from build123d import *

# Parameters (mm, degrees)
F0_W     = 55
F0_H     = 60
F1_DEPTH = 45
F2_W     = 55
F2_H     = 25
F3_DEPTH = 15
F4_W     = 40
F4_H     = 5
F5_DEPTH = 20.001
F7_DEPTH = 45.001
F8_W     = 15
F8_H     = 20
F9_DEPTH = 40


with BuildPart() as f1:
    # F0 (on Top) → F1 (new body)
    with BuildSketch(Plane.XY):
        Rectangle(F0_W, F0_H)
    extrude(amount=F1_DEPTH)

    # F2 (on face) → F3 (cut)
    with BuildSketch(Plane(origin=(0, 30, 0), x_dir=(-1, 0, 0), z_dir=(0, 1, 0))):
        with Locations((0, 32.5)):
            Rectangle(F2_W, F2_H)
    extrude(amount=-F3_DEPTH, mode=Mode.SUBTRACT)

    # F4 (on face) → F5 (cut, through all)
    with BuildSketch(Plane.XY.offset(20)):
        with Locations((-7.5, 17.5)):
            Rectangle(F4_W, F4_H)
    extrude(amount=-F5_DEPTH, mode=Mode.SUBTRACT)

    # F6 (on face) → F7 (cut, through all)
    with BuildSketch(Plane(origin=(0, 15, 0), x_dir=(-1, 0, 0), z_dir=(0, 1, 0))):
        Polygon((-12.5, 45), (-12.5, 20), (-12.5, 0), (27.5, 0), (27.5, 45), align=None)
    extrude(amount=-F7_DEPTH, mode=Mode.SUBTRACT)

    # F8 (on face) → F9 (join)
    with BuildSketch(Plane(origin=(12.5, 0, 0), x_dir=(0, -1, 0), z_dir=(-1, 0, 0))):
        with Locations((22.5, 10)):
            Rectangle(F8_W, F8_H)
    extrude(amount=F9_DEPTH)


solid = f1.part
Could you check a few things on this model? Use its own coordinates, in mm. A direction names the side the tool comes from. Give positions to 0.01 mm unless a question says otherwise; leave off trailing zeros. Loops run counter-clockwise (first coordinate to the right, second up) from the corner with the lowest first, then second, coordinate; pieces in that order, holes last. Notation, with made-up numbers: (46.25, 5) -> (56.25, 5) arc R26 cw to (56.25, 26) -> close; hole circle Ø10 at (68, 62.25). An arc over 180 degrees is marked (long way). Return JSON: item names as keys, results as strings.
Item 1: If we section it at C-C on y = -20: List the corners of the cut face in (x, z) for me.
Geometry results:
{"outline": "(-27.5, 0) -> (27.5, 0) -> (27.5, 45) -> (12.5, 45) -> (12.5, 20) -> (-27.5, 20) -> close"}
Item 2: I need wall thicknesses on L1, parallel to Y at x = -21.5, z = 13; L2, parallel to Y at x = 23.5, z = 33; L3, parallel to Z at x = 15.5, y = 24. Which ranges of each line are inside material? Lowest first, please. Write a range as from..to.
Geometry results:
{"L1": "y = -30..-15, 20..30", "L2": "y = -30..15", "L3": "z = 0..20"}
Item 3: If we section it at A-A on x = -17.5: List the corners of the cut face in (y, z) for me, plus the area to 3 significant figures.
Geometry results:
{"outline": "(-30, 0) -> (-15, 0) -> (-15, 20) -> (-30, 20) -> close; (20, 0) -> (30, 0) -> (30, 20) -> (20, 20) -> close", "area": "500 mm²"}
Item 4: If we section it at D-D on x = 23: List the corners of the cut face in (y, z) for me, plus the area to 4 significant figures.
Geometry results:
{"outline": "(-30, 0) -> (30, 0) -> (30, 20) -> (15, 20) -> (15, 45) -> (-30, 45) -> close", "area": "2,325 mm²"}
Item 5: If we section it at B-B on z = 18: List the corners of the cut face in (x, y) for me.
Geometry results:
{"outline": "(-27.5, -30) -> (27.5, -30) -> (27.5, 30) -> (-27.5, 30) -> (-27.5, 20) -> (12.5, 20) -> (12.5, -15) -> (-27.5, -15) -> close"}
Item 6: We'd pull the mould along Y, two halves only. Please class faces 1 (the flat face through (20, -7, 45)), 2 (the flat face through (6, -30, 17)), 3 (the flat face through (12.5, -5, 23)): +Y half, -Y half, draft (parallel to the pull), parting line (faces both ways), or undercut.
Geometry results:
{"face 1": "draft", "face 2": "-Y half", "face 3": "undercut"}
Item 7: I'm going to push flat-ended pins straight in: pin 1 (12 mm diameter, centred on x = 1, y = 25, fed in from +Z); pin 2 (13.5 mm diameter, centred on y = 6.5, z = 32, fed in from -X); pin 3 (4.5 mm diameter, centred on x = 19.5, z = 31.5, fed in from +Y). Where does each tip first touch, or does it pass through?
Geometry results:
{"pin 1": "stops at z = 20", "pin 2": "stops at x = 12.5", "pin 3": "stops at y = 15"}
Item 8: Which directions (+Z, -Z, +X, -X, +Y, -Y) give clear straight access to the entire face, cutting with the end or side of a thin tool? Please do faces 4 (the flat face through (20, 15, 33)), 5 (the flat face through (-7, -22, 20)), 6 (the flat face through (-7, -15, 10)).
Geometry results:
{"face 4": "+Z, +X, -X, +Y", "face 5": "+Z, -X, +Y, -Y", "face 6": "+Z, -Z, -X"}
